```python
from build123d import *

# Parameters (mm, degrees)
CROQUIS1_R              = 20
CROQUIS1_R_2            = 5
SALIENTE_EXTRUIR1_DEPTH = 15
CROQUIS6_R              = 10
CORTAR_EXTRUIR6_DEPTH   = 5
CROQUIS7_W              = 10
CROQUIS7_H              = 30
CORTAR_EXTRUIR7_DEPTH   = 36
CROQUIS8_W              = 10
CROQUIS8_H              = 20
CORTAR_EXTRUIR9_DEPTH   = 10


with BuildPart() as part:
    # Croquis1 → Saliente-Extruir1 (new, symmetric)
    with BuildSketch(Plane.XY):
        Circle(CROQUIS1_R)
        Circle(CROQUIS1_R_2, mode=Mode.SUBTRACT)
    extrude(amount=SALIENTE_EXTRUIR1_DEPTH, both=True)

    # Croquis6 → Cortar-Extruir6 (cut, symmetric)
    with BuildSketch(Plane.XY):
        Circle(CROQUIS6_R)
    extrude(amount=CORTAR_EXTRUIR6_DEPTH, both=True, mode=Mode.SUBTRACT)

    # Croquis7 → Cortar-Extruir7 (cut)
    with BuildSketch(Plane(origin=(0, 0, 0), x_dir=(0, 0, -1), z_dir=(1, 0, 0))):
        with Locations((0, 5)):
            Rectangle(CROQUIS7_W, CROQUIS7_H)
    extrude(amount=-CORTAR_EXTRUIR7_DEPTH, mode=Mode.SUBTRACT)

    # Croquis8 → Cortar-Extruir9 (cut)
    with BuildSketch(Plane.ZY):
        with Locations((0, 10)):
            Rectangle(CROQUIS8_W, CROQUIS8_H)
    extrude(amount=-CORTAR_EXTRUIR9_DEPTH, mode=Mode.SUBTRACT)


solid = part.part
```
The listing builds one solid part. Answer for the finished solid, in the listing's coordinates (mm). A direction names the side the tool comes from. Coordinates: 2 decimals unless noted, no trailing zeros. Loops run counter-clockwise (first coordinate to the right, second up) from the corner with the lowest first, then second, coordinate; pieces in that order, holes last. Notation, with made-up numbers: (44, 63) -> (73, 63) arc R20 cw to (73, 102) -> close; hole circle Ø11 at (47, -24). An arc over 180 degrees is marked (long way). Return JSON: item names as keys, results as strings. Group by question number.
(1) A cutting plane is placed at C-C on z = -2.5. Write down the section's boundary in (x, y).
(2) A cutting plane is placed at D-D on z = 13.25. Write down the section's boundary in (x, y).
(3) A cutting plane is placed at B-B on y = 6. Write down the section's boundary in (x, z), and give its area (3 significant figures).
(4) Which of the six approach directions +Z, -Z, +X, -X, +Y, -Y give full straight-line access (tool end or side, diameter ignored) to faces 4 (the flat face through (-9, -10, 0)), 5 (the flat face through (4, -4, 15))?
(5) A cutting plane is placed at A-A on x = 1. Write down the section's boundary in (y, z), and give its area (3 significant figures).
(6) Determine the mould class of faces 1 (the flat face through (-5, 5, 5)), 2 (the flat face through (10, 9, 0)), 3 (the cylindrical face through (-1.08, -4.88, 9.93)) for opening direction X: released by +X, released by -X, zero draft, split by the parting line, or undercut.
(7) Given pin 1 Ø5 at (y, z) = (9.5, -1.5) entering from -X; pin 2 Ø6 at (x, z) = (-1.5, 4.5) entering from -Y; pin 3 Ø3 at (x, z) = (12, 8.5) entering from -Y; pin 4 Ø8 at (x, y) = (0, 0) entering from +Z, each flat-ended and moving along its own axis, determine where each tip first touches the part or whether it passes through.
(8) Find the intervals of material crossed by probe 1 along Y at (x, z) = (0, 11); probe 2 along Z at (x, y) = (-10.5, -9); probe 3 along Y at (x, z) = (-10, -0.75), in increasing order. Write a range as from..to.
The answers:
{
 "1": {"outline": "(-17.32, -10) arc R20 ccw (long way) to (10, 17.32) -> (10, 0) arc R10 cw to (0, -10) -> close"},
 "2": {"outline": "circle Ø40 at (0, 0); hole circle Ø10 at (0, 0)"},
 "3": {"outline": "(-19.08, -15) -> (19.08, -15) -> (19.08, 15) -> (-19.08, 15) -> (-19.08, 5) -> (10, 5) -> (10, -5) -> (-19.08, -5) -> close", "area": "854 mm^2"},
 "4": {"face 4": "-X, +Y", "face 5": "+Z, +X, -X, +Y, -Y"},
 "5": {"outline": "(-19.97, -15) -> (-4.9, -15) -> (-4.9, -5) -> (-9.95, -5) -> (-9.95, 5) -> (-4.9, 5) -> (-4.9, 15) -> (-19.97, 15) -> close; (4.9, -15) -> (19.97, -15) -> (19.97, -5) -> (4.9, -5) -> close; (4.9, 5) -> (19.97, 5) -> (19.97, 15) -> (4.9, 15) -> close", "area": "703 mm^2"},
 "6": {"face 1": "zero draft", "face 2": "released by -X", "face 3": "undercut"},
 "7": {"pin 1": "stops at x = 10", "pin 2": "stops at y = -20", "pin 3": "stops at y = -17.02", "pin 4": "passes through"},
 "8": {"probe 1": "y = -20..-5, 5..20", "probe 2": "z = -15..-5, 5..15", "probe 3": "y = -17.32..-10"}
}
